Autodesk Inventor part; units mm, degrees
ref_plane "YZ Plane" through (0, 0, 0) normal (1, 0, 0) x (0, 1, 0)
ref_plane "XZ Plane" through (0, 0, 0) normal (0, 1, 0) x (-1, 0, 0)
ref_plane "XY Plane" through (0, 0, 0) normal (0, 0, 1) x (1, 0, 0)
sketch "Sketch1" plane through (0, 0, 0) normal (0, 1, 0) x (-1, 0, 0)
  line L0 (0, 0) -> (0, -177.8)
  line L1 (0, -177.8) -> (-57.15, -177.8)
  line L2 (0, 0) -> (-57.15, 0)
  line L3 (-57.15, 0) -> (-57.15, -177.8)
  dimension "d0" = 177.8
  dimension "d1" = 57.15
extrude "Extrusion1" add sketch "Sketch1" along normal blind 10
sketch "Sketch2" plane through (0, 10, 0) normal (0, 1, 0) x (1, 0, 0)
  circle A0 centre (28.575, 88.9) radius 3.5
  point P0 (0, 0)
  dimension "d4" = 7
extrude "Extrusion2" cut sketch "Sketch2" against normal through all
pattern_linear "Rectangular Pattern1" count 2 spacing 71.4375 along (0, 0, -1) count 2 spacing 69.85 along (0, 0, 1) of "Extrusion2"
sketch "Sketch3" plane through (0, 10, 0) normal (0, 1, 0) x (1, 0, 0)
  arc A0 (25.1662, 89.6938) -> (31.9838, 89.6937) centre (28.575, 88.9) ccw
  circle A1 centre (28.575, 88.9) radius 6.5
  point P0 (0, 0)
  dimension "d13" = 13
extrude "Extrusion3" cut sketch "Sketch3" against normal blind 5
pattern_linear "Rectangular Pattern2" count 2 spacing 71.4375 along (0, 0, -1) count 2 spacing 69.85 along (0, 0, 1) of "Extrusion3"
sketch "Sketch4" plane through (57.15, 0, 0) normal (1, 0, 0) x (0, 0, -1)
  line L0 (177.8, 0) -> (177.8, 10)
  line L1 (0, 0) -> (177.8, 0)
  line L2 (177.8, 0) -> (177.8, 3)
  line L3 (177.8, 3) -> (0, 3)
  line L4 (0, 3) -> (0, 0)
  dimension "d22" = 3
extrude "Extrusion4" add sketch "Sketch4" along normal blind 50
sketch "Sketch5" plane through (57.15, 3, 0) normal (0, 1, 0) x (1, 0, 0)
  line L0 (50, 177.8) -> (50, 0)
  line L1 (0, 0) -> (0, 177.8)
  line L2 (0, 88.9) -> (8.125, 88.9)
  circle A0 centre (8.125, 88.9) radius 2.125
  point P0 (-57.15, 0)
  dimension "d25" = 8.125
  dimension "d26" = 4.25
extrude "Extrusion5" cut sketch "Sketch5" against normal through all
pattern_linear "Rectangular Pattern3" count 4 spacing 12 along (1, 0, 0) of "Extrusion5"
pattern_linear "Rectangular Pattern4" count 8 spacing 12 along (0, 0, 1) count 8 spacing 12 along (0, 0, -1) of "Extrusion5", "Rectangular Pattern3"
sketch "Sketch6" plane through (0, 10, 0) normal (0, 1, 0) x (1, 0, 0)
  arc A0 (25.1662, 89.6938) -> (31.9838, 89.6937) centre (28.575, 88.9) ccw
  line L0 (28.575, 85.4) -> (28.575, 93.9875)
  arc A1 (31.9838, 89.6937) -> (25.1662, 89.6938) centre (28.575, 90.4875) ccw
  line L1 (35.0264, 89.6938) -> (57.15, 89.6938)
  line L2 (57.15, 0) -> (57.15, 177.8)
  circle A2 centre (46.0882, 89.6938) radius 8
  circle A3 centre (46.0882, 89.6938) radius 10
  point P0 (0, 0)
  dimension "d38" = 16
  dimension "d39" = 20
extrude "Extrusion6" add sketch "Sketch6" along normal blind 17 contours A2 L1 A3 | L1 A3 A2
sketch "Sketch7" plane through (46.0882, 10, -89.6938) normal (0, 1, 0) x (1, 0, 0)
  circle A0 centre (0, 0) radius 8
  line L0 (-8, 0) -> (8, 0)
  point P0 (-46.0882, -89.6938)
sketch "Sketch8" plane through (46.0882, 27, -89.6938) normal (0, 1, 0) x (1, 0, 0)
  point P0 (-46.0882, -89.6938)
properties part number "CraneBaseTest"
Source: CAD feature listing. Evaluate the final solid. Frame: model axes, mm. A direction names the side the tool comes from. Coordinates: 2 decimals unless noted, no trailing zeros. Loops run counter-clockwise (first coordinate to the right, second up) from the corner with the lowest first, then second, coordinate; pieces in that order, holes last. Notation, with made-up numbers: (6, 83) - (24, 83) arc R16 cw to (24, 111) - close; hole circle Ø3 at (-10.5, 19.5). An arc over 180 degrees is marked (long way). One line per item, written item: value. Start each with the question number.
1. Section C-C (x = 48). Return the cut outline in (y, z).
2. Section D-D (y = 13). Return the cut outline in (x, z).
3. Contact query for flat-ended pins moving along their axis: P1, Ø3, axis at x = 15, y = 12.5, coming from the -Z side; P2, Ø1, axis at y = 17.5, z = -87.5, coming from the +X side; P3, Ø5.5, axis at x = 65.275, z = -4.9, coming from the +Y side. Output: stop coordinate, or through.
4. Section A-A (z = -112.9). Return the cut outline in (x, y).
5. Set-up query: faces 1 (the cylindrical face through (31.57, 7.54, -154.57)), 2 (the cylindrical face through (67.3, 1.52, -149.54)). Return all of +Z, -Z, +X, -X, +Y, -Y with unobstructed straight access to the full face (end or side cutting, diameter ignored); none if empty.
6. Mould query, pull axis Z, two halves, no side actions, for faces 3 (the flat face through (0, 5, -88)), 4 (the cylindrical face through (66.256, 1.521, -111.015)). Classes: pulls with the +Z half, pulls with the -Z half, needs draft (parallel to the pull), parting line crosses it, or undercut.
7. Ray query, L1, parallel to X at y = 1.5, z = -40.9; L2, parallel to X at y = 1.3, z = -88.9 (3 decimals); L3, parallel to Y at x = 48, z = -41.5. Return the intervals inside material, ascending.
8. Section B-B (x = 27). Return the cut outline in (y, z), and give its area (3 significant figures).
Verdict:
1. outline: (0, -177.8) - (10, -177.8) - (10, -99.51) - (27, -99.51) - (27, -97.46) - (10, -97.46) - (10, -81.93) - (27, -81.93) - (27, -79.88) - (10, -79.88) - (10, 0) - (0, 0) - close
2. outline: circle Ø20 at (46.09, -89.69); hole circle Ø16 at (46.09, -89.69)
3. P1: passes through
3. P2: stops at x = 55.94
3. P3: stops at y = 3
4. outline: (0, 0) - (63.15, 0) - (63.15, 3) - (57.15, 3) - (57.15, 10) - (0, 10) - close; (67.4, 0) - (75.15, 0) - (75.15, 3) - (67.4, 3) - close; (79.4, 0) - (87.15, 0) - (87.15, 3) - (79.4, 3) - close; (91.4, 0) - (99.15, 0) - (99.15, 3) - (91.4, 3) - close; (103.4, 0) - (107.15, 0) - (107.15, 3) - (103.4, 3) - close
5. face 1: +Y
5. face 2: +Y, -Y
6. face 3: needs draft
6. face 4: undercut
7. L1: x = 0 to 63.15, 67.4 to 75.15, 79.4 to 87.15, 91.4 to 99.15, 103.4 to 107.15
7. L2: x = 0 to 25.075, 32.075 to 63.15, 67.4 to 75.15, 79.4 to 87.15, 91.4 to 99.15, 103.4 to 107.15
7. L3: y = 0 to 10
8. outline: (0, -177.8) - (10, -177.8) - (10, -166.64) - (5, -166.64) - (5, -163.46) - (0, -163.46) - close; (0, -157.21) - (5, -157.21) - (5, -154.03) - (10, -154.03) - (10, -96.79) - (5, -96.79) - (5, -93.61) - (0, -93.61) - close; (0, -85.77) - (5, -85.77) - (5, -82.59) - (10, -82.59) - (10, -25.36) - (5, -25.36) - (5, -22.18) - (0, -22.18) - close; (0, -15.92) - (5, -15.92) - (5, -12.74) - (10, -12.74) - (10, 0) - (0, 0) - close
8. area: 1,480 mm2
